Model file for the job. Use its own axes, mm. A direction names the side the tool comes from. Coordinates: 2 decimals unless noted, no trailing zeros. Loops run counter-clockwise (first coordinate to the right, second up) from the corner with the lowest first, then second, coordinate; pieces in that order, holes last. Notation, with made-up numbers: M 25,73.25 L 56,73.25 A32 ccw 56,110.25 Z; hole C 39.5,7 d1. An arc over 180 degrees is marked long. Write item = value, one per line. Start each with the question number.
from build123d import *

# Parameters (mm, degrees)
DODANIE_WYCI_GNI_CIE1_DEPTH = 5
WYTNIJ_WYCI_GNI_CIE1_DEPTH  = 1
SZKIC3_R                    = 2
WYTNIJ_WYCI_GNI_CIE2_DEPTH  = 5
SZKIC4_R                    = 4
WYTNIJ_WYCI_GNI_CIE3_DEPTH  = 4
SZKIC5_R                    = 5
SZKIC5_R_2                  = 2
DODANIE_WYCI_GNI_CIE2_DEPTH = 5
ZAOKR_GLENIE1_R             = 2


with BuildPart() as part:
    # Szkic1 → Dodanie-wyciągnięcie1 (new body)
    with BuildSketch(Plane.XY):
        with BuildLine():
            Line((-37.935722713, 2.431103393), (-14.066308471, -62.019242173))
            ThreePointArc((-14.066308471, -62.019242173), (0, -71.809734903), (14.066308471, -62.019242173))
            Line((14.066308471, -62.019242173), (37.935722713, 2.431103393))
            ThreePointArc((37.935722713, 2.431103393), (43.929144479, 6.976684311), (50.581769351, 3.465845))
            Line((50.581769351, 3.465845), (51.893527421, 1.164008066))
            ThreePointArc((51.893527421, 1.164008066), (55.268304062, -0.250579595), (57.5, 2.649370209))
            Line((57.5, 2.649370209), (57.5, 14.325924396))
            ThreePointArc((57.5, 14.325924396), (55.449747468, 19.275671864), (50.5, 21.325924396))
            Line((50.5, 21.325924396), (49.5, 21.325924396))
            ThreePointArc((49.5, 21.325924396), (44.550252532, 23.376176928), (42.5, 28.325924396))
            Line((42.5, 28.325924396), (42.5, 95))
            ThreePointArc((42.5, 95), (32.248737342, 119.748737342), (7.5, 130))
            Line((7.5, 130), (-7.5, 130))
            ThreePointArc((-7.5, 130), (-32.248737342, 119.748737342), (-42.5, 95))
            Line((-42.5, 95), (-42.5, 28.325924396))
            ThreePointArc((-42.5, 28.325924396), (-44.550252532, 23.376176928), (-49.5, 21.325924396))
            Line((-49.5, 21.325924396), (-50.5, 21.325924396))
            ThreePointArc((-50.5, 21.325924396), (-55.449747468, 19.275671864), (-57.5, 14.325924396))
            Line((-57.5, 14.325924396), (-57.5, 2.649370209))
            ThreePointArc((-57.5, 2.649370209), (-55.268304062, -0.250579595), (-51.893527421, 1.164008066))
            Line((-51.893527421, 1.164008066), (-50.581769351, 3.465845))
            ThreePointArc((-50.581769351, 3.465845), (-43.929144479, 6.976684311), (-37.935722713, 2.431103393))
        make_face()
    extrude(amount=DODANIE_WYCI_GNI_CIE1_DEPTH)

    # Szkic2 → Wytnij-wyciągnięcie1 (cut)
    with BuildSketch(Plane(origin=(0, 0, 0), x_dir=(-1, 0, 0), z_dir=(0, 0, -1))):
        with BuildLine():
            Line((-27, 78), (27, 78))
            ThreePointArc((27, 78), (29.121320344, 77.121320344), (30, 75))
            Line((30, 75), (30, -9))
            ThreePointArc((30, -9), (29.121320344, -11.121320344), (27, -12))
            Line((27, -12), (-27, -12))
            ThreePointArc((-27, -12), (-29.121320344, -11.121320344), (-30, -9))
            Line((-30, -9), (-30, 75))
            ThreePointArc((-30, 75), (-29.121320344, 77.121320344), (-27, 78))
        make_face()
    extrude(amount=-WYTNIJ_WYCI_GNI_CIE1_DEPTH, mode=Mode.SUBTRACT)

    # Szkic3 → Wytnij-wyciągnięcie2 (cut)
    with BuildSketch(Plane(origin=(0, 0, 0), x_dir=(-1, 0, 0), z_dir=(0, 0, -1))):
        with Locations((-10, 120)):
            Circle(SZKIC3_R)
        with Locations((10, 120)):
            Circle(SZKIC3_R)
    extrude(amount=-WYTNIJ_WYCI_GNI_CIE2_DEPTH, mode=Mode.SUBTRACT)

    # Szkic4 → Wytnij-wyciągnięcie3 (cut)
    with BuildSketch(Plane.XY.offset(5)):
        with Locations((-10, 120)):
            Circle(SZKIC4_R)
        with Locations((10, 120)):
            Circle(SZKIC4_R)
    extrude(amount=-WYTNIJ_WYCI_GNI_CIE3_DEPTH, mode=Mode.SUBTRACT)

    # Szkic5 → Dodanie-wyciągnięcie2 (add)
    with BuildSketch(Plane(origin=(0, 0, 0), x_dir=(-1, 0, 0), z_dir=(0, 0, -1))):
        with Locations((-10, 120)):
            Circle(SZKIC5_R)
        with Locations((-10, 120)):
            Circle(SZKIC5_R_2, mode=Mode.SUBTRACT)
        with Locations((10, 120)):
            Circle(SZKIC5_R)
        with Locations((10, 120)):
            Circle(SZKIC5_R_2, mode=Mode.SUBTRACT)
    extrude(amount=DODANIE_WYCI_GNI_CIE2_DEPTH)

    # Zaokrąglenie1
    zaokr_glenie1_edges = [part.edges().sort_by_distance(p)[0] for p in [
        (15, 120, -5),
        (15, 120, 0),
        (-5, 120, -5),
        (-5, 120, 0),
    ]]
    fillet(zaokr_glenie1_edges, radius=ZAOKR_GLENIE1_R)


solid = part.part
Item 1: Cut at C-C (y = 97.5). Give the cut face in (x, z).
Item 2: Pin check, flat tips, straight feed: pin 1 Ø7 at (x, y) = (10, 120) entering from -Z; pin 2 Ø0.5 at (x, z) = (50, 1.5) entering from +Y; pin 3 Ø5 at (x, z) = (23, -1) entering from +Y; pin 4 Ø5 at (x, y) = (10, 120) entering from +Z. Stop position of each tip, or through.
Item 3: Probe L1, parallel to X at y = 44.5, z = 0.5; L2, parallel to Y at x = 10, z = -2.1; L3, parallel to Y at x = 14, z = -2.5. List the from-to ranges inside material, lowest first.
Item 4: 3-axis set-ups, long thin cutter, end or side, ignore diameter. For faces 1 (the cylindrical face through (-31.975, 120.019, 2.465)), 2 (the cylindrical face through (9.479, 123.966, 3.028)), 3 (the flat face through (42.5, 61, 2)): which of +Z, -Z, +X, -X, +Y, -Y reach the whole face in a straight line?
Item 5: Pull direction Y, two halves, no side cores. Call faces 4 (the cylindrical face through (43.818, 6.967, 2.465)), 5 (the flat face through (8, 119, 1)), 6 (the cylindrical face through (5.23, 121.5, -2.49)): +Y half, -Y half, draft (parallel to the pull), parting line (faces both ways), or undercut.
Item 6: Cut at D-D (x = -33.5). Give the cut face in (y, z).
Item 7: Cut at A-A (x = -10). Give the cut face in (y, z).
Item 8: Cut at B-B (y = 120). Give the number of separate pieces and of enclosed holes in the cut face, plus the area to 3 significant figures.
Reported:
q1.outline = M -42.41,0 L 42.41,0 L 42.41,5 L -42.41,5 Z
q2.pin_1 = -5
q2.pin_2 = 21.33
q2.pin_3 = 127.41
q2.pin_4 = 1
q3.L1 = -42.5 to -30, 30 to 42.5
q3.L2 = 115 to 118, 122 to 125
q3.L3 = 117 to 123
q4.face_1 = +Z, -Z, -X, +Y
q4.face_2 = +Z
q4.face_3 = +Z, -Z, +X, +Y
q5.face_4 = -Y half
q5.face_5 = undercut
q5.face_6 = parting line
q6.outline = M -9.55,0 L 118.43,0 L 118.43,5 L -9.55,5 Z
q7.outline = M -67.99,0 L -12,0 L -12,1 L 78,1 L 78,0 L 113,0 A2 cw 115,-2 L 115,-3 A2 ccw 117,-5 L 118,-5 L 118,1 L 116,1 L 116,5 L -67.99,5 Z; M 122,-5 L 123,-5 A2 ccw 125,-3 L 125,-2 A2 cw 127,0 L 129.91,0 L 129.91,5 L 124,5 L 124,1 L 122,1 Z
q8.separate_pieces = 3
q8.enclosed_holes = 0
q8.area = 308 mm^2
